Work out the finished part from the listing and answer in its coordinate system (mm). A direction names the side the tool comes from. Coordinates: 2 decimals unless noted, no trailing zeros. Order: outer loops, then holes, each group sorted by start corner. A loop starts at its lowest first (then second) coordinate and runs counter-clockwise, first axis right, second up. Notation, with made-up numbers: M 19,56 L 76,56 A19 ccw 76,72 Z; hole C 36.5,81 d3. An arc over 180 degrees is marked long. Answer in a Markdown table with one row per item. Add a question column.
Item 1: The part is cut by section B-B (z = 16). Write down the section's boundary in (x, y).
Item 2: The part is cut by section A-A (y = 4). Write down the section's boundary in (x, z).
Item 3: Which of the six approach directions +Z, -Z, +X, -X, +Y, -Y give full straight-line access (tool end or side, diameter ignored) to faces 1 (the face through (0, 4, 25.25)), 2 (the face through (25.25, 5, -2)), 3 (the face through (-19.25, 5, -27)), 4 (the face through (0, 8, -22.25))?
Item 4: The part is cut by section C-C (x = -32.25). Write down the section's boundary in (y, z).
Item 5: The mould has two halves that part along X. Classify faces 5 (the face through (0, 4, -25.25)), 6 (the face through (0, 2.3, -27)), 7 (the face through (36.25, 5, 0)), 8 (the face through (0, 8, 22.25)): released by +X, released by -X, zero draft, split by the parting line, or undercut.
Item 6: The part is cut by section D-D (z = 24.25). Write down the section's boundary in (x, y).
Item 7: Flat-ended cylindrical pins translate along their axes: pin 1 Ø2.5 at (x, z) = (32.25, -24.25) entering from +Y; pin 2 Ø2 at (x, y) = (-22.5, 7.5) entering from -Z. Find the tip coordinate at first contact, or state that the pin passes through.
Item 8: Consider line 1 (Z direction, x = -32, y = 6.75); line 2 (X direction, y = 6, z = 24.25); line 3 (X direction, y = 5, z = 0). Determine where each line is inside the solid, lowest interval first. Write a range as from..to.
from build123d import *

# Parameters (mm, degrees)
SKETCH1_W           = 56.5
SKETCH1_H           = 56.5
SKETCH1_W_2         = 50.5
SKETCH1_H_2         = 50.5
SKETCH1_R           = 1.65
BOSS_EXTRUDE1_DEPTH = 8.6
SKETCH2_W           = 50.5
SKETCH2_H           = 50.5
SKETCH2_W_2         = 44.5
SKETCH2_H_2         = 44.5
BOSS_EXTRUDE2_DEPTH = 2
BOSS_EXTRUDE3_START = 6.6
SKETCH4_W           = 50.5
SKETCH4_H           = 50.5
SKETCH4_W_2         = 44.5
SKETCH4_H_2         = 44.5
BOSS_EXTRUDE3_DEPTH = 2
CUT_EXTRUDE1_START  = 2
SKETCH5_W           = 6
SKETCH5_H           = 17.961455198
CUT_EXTRUDE1_DEPTH  = 4.6
SKETCH6_W           = 87.3205389
SKETCH6_H           = 82.15723747
CUT_EXTRUDE2_DEPTH  = 2.3
CUT_EXTRUDE4_DEPTH  = 10
SKETCH8_W           = 8
SKETCH8_H           = 40.5
BOSS_EXTRUDE4_DEPTH = 6.3
SKETCH9_W           = 6
SKETCH9_H           = 6.3
CUT_EXTRUDE5_DEPTH  = 4


with BuildPart() as part:
    # Sketch1 → Boss-Extrude1 (new body)
    with BuildSketch(Plane(origin=(0, 0, 0), x_dir=(1, 0, 0), z_dir=(0, 1, 0))):
        Rectangle(SKETCH1_W, SKETCH1_H)
        Rectangle(SKETCH1_W_2, SKETCH1_H_2, mode=Mode.SUBTRACT)
        Polygon((-28.25, -28.25), (-28.25, -12.25), (-36.25, -20.25), (-36.25, -30.25), (-32.25, -34.25), (-24.25, -34.25), (-18.25, -28.25), align=None)
        with Locations((-32.25, -24.25)):
            Circle(SKETCH1_R, mode=Mode.SUBTRACT)
        Polygon((28.25, -28.25), (18.25, -28.25), (24.25, -34.25), (32.25, -34.25), (36.25, -30.25), (36.25, -20.25), (28.25, -12.25), align=None)
        with Locations((32.25, -24.25)):
            Circle(SKETCH1_R, mode=Mode.SUBTRACT)
        Polygon((24.25, 34.25), (18.25, 28.25), (28.25, 28.25), (28.25, 12.25), (36.25, 20.25), (36.25, 30.25), (32.25, 34.25), align=None)
        with Locations((32.25, 24.25)):
            Circle(SKETCH1_R, mode=Mode.SUBTRACT)
        Polygon((-36.25, 20.25), (-28.25, 12.25), (-28.25, 28.25), (-18.25, 28.25), (-24.25, 34.25), (-32.25, 34.25), (-36.25, 30.25), align=None)
        with Locations((-32.25, 24.25)):
            Circle(SKETCH1_R, mode=Mode.SUBTRACT)
    extrude(amount=BOSS_EXTRUDE1_DEPTH)

    # Sketch2 → Boss-Extrude2 (add)
    with BuildSketch(Plane(origin=(0, 0, 0), x_dir=(1, 0, 0), z_dir=(0, 1, 0))):
        Rectangle(SKETCH2_W, SKETCH2_H)
        Rectangle(SKETCH2_W_2, SKETCH2_H_2, mode=Mode.SUBTRACT)
    extrude(amount=BOSS_EXTRUDE2_DEPTH)

    # Sketch4 → Boss-Extrude3 (add)
    with BuildSketch(Plane(origin=(0, 0, 0), x_dir=(1, 0, 0), z_dir=(0, 1, 0)).offset(BOSS_EXTRUDE3_START)):
        Rectangle(SKETCH4_W, SKETCH4_H)
        Rectangle(SKETCH4_W_2, SKETCH4_H_2, mode=Mode.SUBTRACT)
    extrude(amount=BOSS_EXTRUDE3_DEPTH)

    # Sketch5 → Cut-Extrude1 (cut)
    with BuildSketch(Plane(origin=(0, 0, 0), x_dir=(1, 0, 0), z_dir=(0, 1, 0)).offset(CUT_EXTRUDE1_START)):
        with Locations((-22.25, 28.869783692)):
            Rectangle(SKETCH5_W, SKETCH5_H)
        with Locations((22.25, 28.869783692)):
            Rectangle(SKETCH5_W, SKETCH5_H)
    extrude(amount=CUT_EXTRUDE1_DEPTH, mode=Mode.SUBTRACT)

    # Sketch6 → Cut-Extrude2 (cut)
    with BuildSketch(Plane.XZ):
        with Locations((1.898272585, -1.518618068)):
            Rectangle(SKETCH6_W, SKETCH6_H)
    extrude(amount=-CUT_EXTRUDE2_DEPTH, mode=Mode.SUBTRACT)

    # Sketch7 → Cut-Extrude4 (cut)
    with BuildSketch(Plane(origin=(0, 8.6, 0), x_dir=(1, 0, 0), z_dir=(0, 1, 0))):
        Polygon((-36.25, -30.25), (-36.25, -28.25), (-40.881768663, -28.25), (-40.881768663, -34.995320637), (0, -34.995320637), (0, -28.25), (-18.25, -28.25), (-24.25, -34.25), (-32.25, -34.25), align=None)
        Polygon((18.25, -28.25), (0, -28.25), (0, -34.995320637), (39.184342226, -34.995320637), (39.184342226, -28.25), (36.25, -28.25), (36.25, -30.25), (32.25, -34.25), (24.25, -34.25), align=None)
        Polygon((36.25, 20.25), (36.25, -20.25), (28.25, -12.25), (28.25, 12.25), align=None)
        Polygon((-36.25, 20.25), (-36.25, -20.25), (-28.25, -12.25), (-28.25, 12.25), align=None)
        Polygon((-36.25, 30.25), (-36.25, 28.25), (-18.25, 28.25), (-24.25, 34.25), (-32.25, 34.25), align=None)
        Polygon((-38.207606214, 28.25), (-36.25, 28.25), (-36.25, 30.25), (-32.25, 34.25), (-24.25, 34.25), (-18.25, 28.25), (0, 28.25), (0, 36.724555445), (-38.207606214, 36.724555445), align=None)
        Polygon((28.25, 12.25), (36.25, 20.25), (28.25, 20.25), align=None)
        Polygon((28.25, -20.25), (36.25, -20.25), (28.25, -12.25), align=None)
        Polygon((-18.25, -28.25), (-36.25, -28.25), (-36.25, -30.25), (-32.25, -34.25), (-24.25, -34.25), align=None)
        Polygon((-28.25, -12.25), (-36.25, -20.25), (-28.25, -20.25), align=None)
        Polygon((-28.25, 20.25), (-36.25, 20.25), (-28.25, 12.25), align=None)
        Polygon((24.25, 34.25), (18.25, 28.25), (36.25, 28.25), (36.25, 30.25), (32.25, 34.25), align=None)
        Polygon((0, 36.724555445), (0, 28.25), (18.25, 28.25), (24.25, 34.25), (32.25, 34.25), (36.25, 30.25), (36.25, 28.25), (40.981198071, 28.25), (40.981198071, 36.724555445), align=None)
        Polygon((36.25, -28.25), (18.25, -28.25), (24.25, -34.25), (32.25, -34.25), (36.25, -30.25), align=None)
    extrude(amount=-CUT_EXTRUDE4_DEPTH, mode=Mode.SUBTRACT)

    # Sketch8 → Boss-Extrude4 (add)
    with BuildSketch(Plane(origin=(0, 8.6, 0), x_dir=(1, 0, 0), z_dir=(0, 1, 0))):
        with Locations((-32.25, 0)):
            Rectangle(SKETCH8_W, SKETCH8_H)
        with Locations((32.25, 0)):
            Rectangle(SKETCH8_W, SKETCH8_H)
    extrude(amount=-BOSS_EXTRUDE4_DEPTH)

    # Sketch9 → Cut-Extrude5 (cut)
    with BuildSketch(Plane(origin=(0, 0, -28.25), x_dir=(-1, 0, 0), z_dir=(0, 0, -1))):
        with Locations((-22.25, 5.45)):
            Rectangle(SKETCH9_W, SKETCH9_H)
        with Locations((22.25, 5.45)):
            Rectangle(SKETCH9_W, SKETCH9_H)
    extrude(amount=-CUT_EXTRUDE5_DEPTH, mode=Mode.SUBTRACT)


solid = part.part
Reply:
| question | item | result |
|---|---|---|
| 1 | outline | M -36.25,2.3 L -25.25,2.3 L -25.25,6.6 L -22.25,6.6 L -22.25,8.6 L -36.25,8.6 Z; M 22.25,6.6 L 25.25,6.6 L 25.25,2.3 L 36.25,2.3 L 36.25,8.6 L 22.25,8.6 Z |
| 2 | outline | M -36.25,-28.25 L -25.25,-28.25 L -25.25,25.25 L 25.25,25.25 L 25.25,-28.25 L 36.25,-28.25 L 36.25,28.25 L -36.25,28.25 Z; M -19.25,-28.25 L 19.25,-28.25 L 19.25,-25.25 L -19.25,-25.25 Z; hole C -32.25,-24.25 d3.3; hole C -32.25,24.25 d3.3; hole C 32.25,-24.25 d3.3; hole C 32.25,24.25 d3.3 |
| 3 | face 1 | -Y |
| 3 | face 2 | -Z, -Y |
| 3 | face 3 | -Z, +Y, -Y |
| 3 | face 4 | +Y, -Y |
| 4 | outline | M 2.3,-28.25 L 8.6,-28.25 L 8.6,-25.9 L 2.3,-25.9 Z; M 2.3,-22.6 L 8.6,-22.6 L 8.6,22.6 L 2.3,22.6 Z; M 2.3,25.9 L 8.6,25.9 L 8.6,28.25 L 2.3,28.25 Z |
| 5 | face 5 | undercut |
| 5 | face 6 | zero draft |
| 5 | face 7 | released by +X |
| 5 | face 8 | undercut |
| 6 | outline | M -36.25,2.3 L -33.9,2.3 L -33.9,8.6 L -36.25,8.6 Z; M -30.6,2.3 L -25.25,2.3 L -25.25,6.6 L 25.25,6.6 L 25.25,2.3 L 30.6,2.3 L 30.6,8.6 L -30.6,8.6 Z; M 33.9,2.3 L 36.25,2.3 L 36.25,8.6 L 33.9,8.6 Z |
| 7 | pin 1 | passes through |
| 7 | pin 2 | stops at z = -24.25 |
| 8 | line 1 | z = -28.25..-25.88, -22.62..22.62, 25.88..28.25 |
| 8 | line 2 | x = -36.25..-33.9, -30.6..-25.25, 25.25..30.6, 33.9..36.25 |
| 8 | line 3 | x = -36.25..-25.25, 25.25..36.25 |
